from build123d import *

# Parameters (mm, degrees)
ESQUISSE1_W             = 95.08
ESQUISSE1_H             = 114.3
ESQUISSE1_R             = 1
ESQUISSE1_W_2           = 3
ESQUISSE1_H_2           = 6
BOSS_EXTRU_1_DEPTH      = 4
ESQUISSE2_R             = 1
ENL_V_MAT_EXTRU_1_DEPTH = 10
ENL_V_START             = -10
ESQUISSE3_R             = 1
ENL_V_MAT_EXTRU_2_DEPTH = 10
CONG_1_R                = 3


with BuildPart() as part:
    # Esquisse1 → Boss.-Extru.1 (new body)
    with BuildSketch(Plane(origin=(0, 0, 0), x_dir=(1, 0, 0), z_dir=(0, 1, 0))):
        Rectangle(ESQUISSE1_W, ESQUISSE1_H)
        with Locations(Location((-39.54, -9, 0), (0, 0, 270))):
            Circle(ESQUISSE1_R, mode=Mode.SUBTRACT)
        with Locations(Location((-0.42, -9, 0), (0, 0, 270))):
            Circle(ESQUISSE1_R, mode=Mode.SUBTRACT)
        with Locations(Location((-0.42, 9, 0), (0, 0, 90))):
            Circle(ESQUISSE1_R, mode=Mode.SUBTRACT)
        with Locations(Location((-39.54, 9, 0), (0, 0, 90))):
            Circle(ESQUISSE1_R, mode=Mode.SUBTRACT)
        with Locations((41.54, 0)):
            Rectangle(ESQUISSE1_W_2, ESQUISSE1_H_2, mode=Mode.SUBTRACT)
        with Locations((41.54, -50)):
            Rectangle(ESQUISSE1_W_2, ESQUISSE1_H_2, mode=Mode.SUBTRACT)
        with Locations((41.54, 50)):
            Rectangle(ESQUISSE1_W_2, ESQUISSE1_H_2, mode=Mode.SUBTRACT)
        with Locations((-41.54, -50)):
            Rectangle(ESQUISSE1_W_2, ESQUISSE1_H_2, mode=Mode.SUBTRACT)
        with Locations((-41.54, 50)):
            Rectangle(ESQUISSE1_W_2, ESQUISSE1_H_2, mode=Mode.SUBTRACT)
        with Locations((-41.54, 0)):
            Rectangle(ESQUISSE1_W_2, ESQUISSE1_H_2, mode=Mode.SUBTRACT)
    extrude(amount=BOSS_EXTRU_1_DEPTH)

    # Esquisse2 → Enlèv. mat.-Extru.1 (cut)
    with BuildSketch(Plane.ZY.offset(47.54)):
        with Locations((-50, 2)):
            Circle(ESQUISSE2_R)
        with Locations((0, 2)):
            Circle(ESQUISSE2_R)
        with Locations((50, 2)):
            Circle(ESQUISSE2_R)
    extrude(amount=-ENL_V_MAT_EXTRU_1_DEPTH, mode=Mode.SUBTRACT)

    # Esquisse3 → Enlèv. mat.-Extru.2 (cut)
    with BuildSketch(Plane(origin=(47.54, 0, 0), x_dir=(0, 0, -1), z_dir=(1, 0, 0)).offset(ENL_V_START)):
        with Locations(Location((-50, 2, 0), (0, 0, 180))):
            Circle(ESQUISSE3_R)
        with Locations(Location((0, 2, 0), (0, 0, 180))):
            Circle(ESQUISSE3_R)
        with Locations(Location((50, 2, 0), (0, 0, 180))):
            Circle(ESQUISSE3_R)
    extrude(amount=ENL_V_MAT_EXTRU_2_DEPTH, mode=Mode.SUBTRACT)

    # Congé1
    cong_1_edges = [part.edges().sort_by_distance(p)[0] for p in [
        (0, 4, 57.15),
        (0, 4, -57.15),
    ]]
    fillet(cong_1_edges, radius=CONG_1_R)


solid = part.part
CAD build for the part. Positions are in the model's coordinates, mm. Give positions to 0.01 mm unless a question says otherwise; leave off trailing zeros. Put each result on its own line as item: value. Start each with the question number.
(1) Band-saw the part on A-A, the plane y = 2. Give the number of separate pieces and of enclosed holes in the cut face, and give its area (3 significant figures).
(2) Flat gauge pins, fed straight in: pin 1 Ø0.6 at (y, z) = (2.5, 50) entering from -X; pin 2 Ø1.8 at (y, z) = (2, 50) entering from +X; pin 3 Ø0.9 at (x, y) = (-41, 2) entering from +Z. Where does each tip first touch, or does it go through?
(3) Mould opens along Z. For faces 1 (the face through (-43.04, 3, -1)), 2 (the face through (0.67, 3.14, -56.25)) say: +Z half, -Z half, draft (parallel to the pull), parting line (faces both ways), or undercut.
(4) Probe L1, parallel to X at y = 1.9, z = -52; L2, parallel to Y at x = -46.55, z = 0; L3, parallel to Z at x = 38.15, y = 2. List the from-to ranges inside material, lowest first.
Response values:
1. separate pieces: 1
1. enclosed holes: 4
1. area: 10,600 mm2
2. pin 1: stops at x = -37.54
2. pin 2: stops at x = 37.54
2. pin 3: stops at z = 57.1
3. face 1: undercut
3. face 2: -Z half
4. L1: x = -47.54 to -43.04, -40.04 to 40.04, 43.04 to 47.54
4. L2: y = 0 to 1, 3 to 4
4. L3: z = -56.98 to -51, -49 to -1, 1 to 49, 51 to 56.98
